Read the model definition and answer for the solid it produces. Units are mm, in the model's axes. Coordinates: 2 decimals unless noted, no trailing zeros. Loops run counter-clockwise (first coordinate to the right, second up) from the corner with the lowest first, then second, coordinate; pieces in that order, holes last. Notation, with made-up numbers: (35.25, -29.5) -> (43.25, -29.5) arc R26 ccw to (43.25, -15.5) -> close; hole circle Ø11 at (-30, 77.5). An arc over 180 degrees is marked (long way). Answer as a JSON object with one key per item and string values. Group by question number.
Q1. Straight lines are drawn through the part: line 1 along Y through (x, z) = (0.25, 24.5); line 2 along Z through (x, y) = (1.75, 3). For each, find the intervals that lie inside material, in ascending order. Write a range as [from, to].
Q2. The part is cut by section B-B on x = 0. Write down the section's boundary in (y, z), and give its area (3 significant figures).
Q3. This flat-tipped pin is pushed along its axis until it touches: P1, Ø3.5, axis at x = -3, z = 6, coming from the -Y side. Where does it stop, or does it pass through?
Q4. The part is cut by section C-C on z = 27.5. Write down the section's boundary in (x, y) (1 decimal).
Q5. The part is cut by section A-A on y = 7.25. Write down the section's boundary in (x, z).
from build123d import *

# Parameters (mm, degrees)
F1_DEPTH = 38.1
F3_D     = 4.2333333333
F4_W     = 19.3675
F4_H     = 38.1
F5_DEPTH = 12.7
F6_R     = 3.175


with BuildPart() as f1:
    # F0 (on Top) → F1 (new body, symmetric)
    with BuildSketch(Plane.XY):
        with BuildLine():
            Line((-0.9525, 4.0160926284), (-0.9525, 24.4475))
            Line((-0.9525, 24.4475), (-4.1275, 24.4475))
            Line((-4.1275, 24.4475), (-4.1275, 0))
            ThreePointArc((-4.1275, 0), (3.2378773911, -2.5597668351), (-0.9525, 4.0160926284))
        make_face()
    extrude(amount=F1_DEPTH, both=True)

    # F3 (through all)
    with Locations(Plane.XY.offset(38.1)):
        with Locations((0, 0)):
            Hole(F3_D / 2)

    # F4 (on face) → F5 (cut, symmetric)
    with BuildSketch(Plane.YZ.offset(-0.9525)):
        with Locations((5.55625, 0)):
            Rectangle(F4_W, F4_H)
    extrude(amount=F5_DEPTH, both=True, mode=Mode.SUBTRACT)

    # F6
    f6_edges = [f1.edges().sort_by_distance(p)[0] for p in [
        (-2.54, 15.24, 19.05),
        (-2.54, 15.24, -19.05),
    ]]
    fillet(f6_edges, radius=F6_R)


solid = f1.part
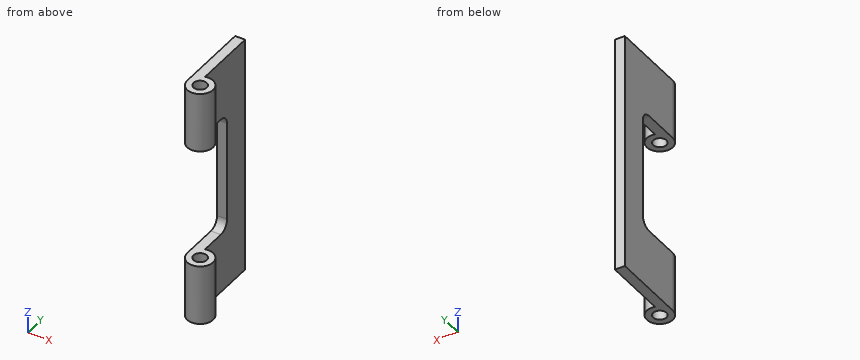
Final values:
{
 "1": {"line 1": "y = [-4.12, -2.1], [2.1, 4.12]", "line 2": "z = [-38.1, -19.05], [19.05, 38.1]"},
 "2": {"outline": "(-4.13, -38.1) -> (-2.12, -38.1) -> (-2.12, -19.05) -> (-4.13, -19.05) -> close; (-4.13, 19.05) -> (-2.12, 19.05) -> (-2.12, 38.1) -> (-4.13, 38.1) -> close; (2.12, -38.1) -> (4.13, -38.1) -> (4.13, -19.05) -> (2.12, -19.05) -> close; (2.12, 19.05) -> (4.13, 19.05) -> (4.13, 38.1) -> (2.12, 38.1) -> close", "area": "153 mm2"},
 "3": {"P1": "stops at y = 15.24"},
 "4": {"outline": "(-4.1, 0) arc R4.1 ccw (long way) to (-1, 4) -> (-1, 24.4) -> (-4.1, 24.4) -> close; hole circle Ø4.2 at (0, 0)"},
 "5": {"outline": "(-4.13, -38.1) -> (-0.95, -38.1) -> (-0.95, -19.05) -> (-4.13, -19.05) -> close; (-4.13, 19.05) -> (-0.95, 19.05) -> (-0.95, 38.1) -> (-4.13, 38.1) -> close"}
}
